Verification items for the finished model (mm, model axes). A direction names the side the tool comes from. Coordinates: 2 decimals unless noted, no trailing zeros. Order: outer loops, then holes, each group sorted by start corner. A loop starts at its lowest first (then second) coordinate and runs counter-clockwise, first axis right, second up. Notation, with made-up numbers: (45.25, -9.5) -> (50.25, -9.5) arc R33 cw to (50.25, 29.5) -> close; hole circle Ø5 at (57, 9.25). An arc over 180 degrees is marked (long way). Write item = value, one per line. Start each with the question number.
from build123d import *

# Parameters (mm, degrees)
SKETCH1_W           = 13.5
SKETCH1_H           = 14.5
BOSS_EXTRUDE1_DEPTH = 17
SKETCH2_W           = 15
SKETCH2_H           = 16
BOSS_EXTRUDE2_DEPTH = 1
SKETCH3_W           = 12
SKETCH3_H           = 4.5
CUT_EXTRUDE1_DEPTH  = 10


with BuildPart() as part:
    # Sketch1 → Boss-Extrude1 (new body)
    with BuildSketch(Plane.XY):
        Rectangle(SKETCH1_W, SKETCH1_H)
    extrude(amount=BOSS_EXTRUDE1_DEPTH)

    # Sketch2 → Boss-Extrude2 (add)
    with BuildSketch(Plane.XY):
        Rectangle(SKETCH2_W, SKETCH2_H)
    extrude(amount=-BOSS_EXTRUDE2_DEPTH)

    # Sketch3 → Cut-Extrude1 (cut)
    with BuildSketch(Plane(origin=(0, 0, -1), x_dir=(-1, 0, 0), z_dir=(0, 0, -1))):
        with Locations((0, 4)):
            Rectangle(SKETCH3_W, SKETCH3_H)
        with Locations((0, -4)):
            Rectangle(SKETCH3_W, SKETCH3_H)
    extrude(amount=-CUT_EXTRUDE1_DEPTH, mode=Mode.SUBTRACT)


solid = part.part
Item 1: Section check B-B (y = -7). Record the boundary of the cut face in (x, z).
Item 2: Section check C-C (x = 2). Record the boundary of the cut face in (y, z).
Item 3: Tool access check on faces 4 (the flat face through (0, -7.25, 8)), 5 (the flat face through (-6, -4, 4)), 6 (the flat face through (0, 7.25, 8)). Record the directions out of +Z, -Z, +X, -X, +Y, -Y that give a thin tool (end or side, any length) a straight path to the whole face; none if there is none.
Item 4: Gauge pin test, flat ends, axial feed: P1, Ø3, axis at x = 0.5, z = 2, coming from the -Y side; P2, Ø1.5, axis at y = -2.5, z = 13, coming from the -X side; P3, Ø5, axis at x = -3.5, z = 14, coming from the +Y side. Record the tip position at first contact, or that the pin passes through.
Item 5: Thickness scan on line 1 (Y direction, x = 3, z = 8); line 2 (X direction, y = 2.75, z = 4); line 3 (Y direction, x = -4.5, z = 12). Record the ranges inside material, lowest first.
Item 6: Section check A-A (z = 7). Record the boundary of the cut face in (x, y), then the cut area to 4 significant figures.
Item 7: Mould release check, pull along Y, two halves, no side actions. Record for faces 1 (the flat face through (-7, 0, 0)), 2 (the flat face through (-0.1, -8, -0.5)), 3 (the flat face through (0, 6.25, 4)): pulls with the +Y half, pulls with the -Y half, needs draft (parallel to the pull), parting line crosses it, or undercut.
Item 8: Section check D-D (z = 10.25). Record the boundary of the cut face in (x, y).
Filled sheet:
q1.outline = (-7.5, -1) -> (7.5, -1) -> (7.5, 0) -> (6.75, 0) -> (6.75, 17) -> (-6.75, 17) -> (-6.75, 0) -> (-7.5, 0) -> close
q2.outline = (-8, -1) -> (-6.25, -1) -> (-6.25, 9) -> (-1.75, 9) -> (-1.75, -1) -> (1.75, -1) -> (1.75, 9) -> (6.25, 9) -> (6.25, -1) -> (8, -1) -> (8, 0) -> (7.25, 0) -> (7.25, 17) -> (-7.25, 17) -> (-7.25, 0) -> (-8, 0) -> close
q3.face_4 = +Z, +X, -X, -Y
q3.face_5 = -Z
q3.face_6 = +Z, +X, -X, +Y
q4.P1 = -7.25
q4.P2 = -6.75
q4.P3 = 7.25
q5.line_1 = -7.25 to -6.25, -1.75 to 1.75, 6.25 to 7.25
q5.line_2 = -6.75 to -6, 6 to 6.75
q5.line_3 = -7.25 to 7.25
q6.outline = (-6.75, -7.25) -> (6.75, -7.25) -> (6.75, 7.25) -> (-6.75, 7.25) -> close; hole (-6, -6.25) -> (6, -6.25) -> (6, -1.75) -> (-6, -1.75) -> close; hole (-6, 1.75) -> (6, 1.75) -> (6, 6.25) -> (-6, 6.25) -> close
q6.area = 87.75 mm^2
q7.face_1 = needs draft
q7.face_2 = pulls with the -Y half
q7.face_3 = undercut
q8.outline = (-6.75, -7.25) -> (6.75, -7.25) -> (6.75, 7.25) -> (-6.75, 7.25) -> close
